```python
from build123d import *

# Parameters (mm, degrees)
SKETCH1_W           = 24.5
SKETCH1_H           = 13.110526316
SKETCH1_W_2         = 23.5
SKETCH1_H_2         = 10
BOSS_EXTRUDE1_DEPTH = 6
BOSS_EXTRUDE2_DEPTH = 6
SKETCH3_W           = 13.982681085
SKETCH3_H           = 4.437803864
CUT_EXTRUDE1_DEPTH  = 11
SKETCH4_W           = 0.982681085
SKETCH4_H           = 2.509369157
BOSS_EXTRUDE3_DEPTH = 6
SKETCH5_W           = 4.892282449
SKETCH5_H           = 6
BOSS_EXTRUDE4_DEPTH = 3.3
FILLET1_R           = 1.5
SKETCH6_W           = 3.982650634
SKETCH6_H           = 6.804776745
CUT_EXTRUDE2_DEPTH  = 10


with BuildPart() as part:
    # Sketch1 → Boss-Extrude1 (new body)
    with BuildSketch(Plane(origin=(0, 0, 0), x_dir=(1, 0, 0), z_dir=(0, 1, 0))):
        with Locations((-3.853684211, 3.800526316)):
            Rectangle(SKETCH1_W, SKETCH1_H)
        with Locations((-3.853684211, 3.855789474)):
            Rectangle(SKETCH1_W_2, SKETCH1_H_2, mode=Mode.SUBTRACT)
    extrude(amount=BOSS_EXTRUDE1_DEPTH)

    # Sketch2 → Boss-Extrude2 (add)
    with BuildSketch(Plane(origin=(0, 6, 0), x_dir=(1, 0, 0), z_dir=(0, 1, 0))):
        Polygon((-10.353684211, 10.355789474), (-10.353684211, 15.855789474), (2.646315789, 15.855789474), (2.646315789, 10.355789474), (4.146315789, 10.355789474), (4.146315789, 17.610127639), (-11.853684211, 17.610127639), (-11.853684211, 10.355789474), align=None)
    extrude(amount=-BOSS_EXTRUDE2_DEPTH)

    # Sketch3 → Cut-Extrude1 (cut)
    with BuildSketch(Plane(origin=(0, 6, 0), x_dir=(1, 0, 0), z_dir=(0, 1, 0))):
        with Locations((-3.362343669, 9.146256699)):
            Rectangle(SKETCH3_W, SKETCH3_H)
    extrude(amount=-CUT_EXTRUDE1_DEPTH, mode=Mode.SUBTRACT)

    # Sketch4 → Boss-Extrude3 (add)
    with BuildSketch(Plane(origin=(0, 6, 0), x_dir=(1, 0, 0), z_dir=(0, 1, 0))):
        with Locations((3.137656332, 10.110474052)):
            Rectangle(SKETCH4_W, SKETCH4_H)
    extrude(amount=-BOSS_EXTRUDE3_DEPTH)

    # Sketch5 → Boss-Extrude4 (add)
    with BuildSketch(Plane(origin=(8.396315789, 0, 0), x_dir=(0, 0, -1), z_dir=(1, 0, 0))):
        with Locations((7.90964825, 3)):
            Rectangle(SKETCH5_W, SKETCH5_H)
    extrude(amount=BOSS_EXTRUDE4_DEPTH)

    # Fillet1
    fillet1_edges = [part.edges().sort_by_distance(p)[0] for p in [
        (8.396315789, 3, -5.463507025),
    ]]
    fillet(fillet1_edges, radius=FILLET1_R)

    # Sketch6 → Cut-Extrude2 (cut)
    with BuildSketch(Plane(origin=(0, 6, 0), x_dir=(1, 0, 0), z_dir=(0, 1, 0))):
        with Locations((10.294706848, 7.545396136)):
            Rectangle(SKETCH6_W, SKETCH6_H)
    extrude(amount=-CUT_EXTRUDE2_DEPTH, mode=Mode.SUBTRACT)


solid = part.part
```
Check sheet for the modelled part. Datum: model origin and axes. Units: mm. A direction names the side the tool comes from. Coordinates: 2 decimals unless noted, no trailing zeros. Write each loop counter-clockwise with the first axis right and the second up, starting at its lowest first coordinate (ties: lowest second). Pieces come first, ordered by that corner, then holes. Notation, with made-up numbers: M -22,68.25 L 25,68.25 A26 cw 25,105.25 Z; hole C 58,47.5 d4. An arc over 180 degrees is marked long. Write item = value, one per line. Start each with the question number.
1. Go/stop test with flat-tipped pins: pin 1 (1.8 mm diameter, centred on y = 1.5, z = -6.5, fed in from +X); pin 2 (1.2 mm diameter, centred on x = 5.5, y = 2, fed in from -Z); pin 3 (3 mm diameter, centred on y = 2, z = 0.5, fed in from +X). Record where each tip stops, or that it passes through.
2. Mould release check, pull along X, two halves, no side actions. Record for faces 4 (the flat face through (-16.104, 3, -4)), 5 (the flat face through (-15.604, 3, -4)), 6 (the flat face through (6, 3, -10.356)): pulls with the +X half, pulls with the -X half, needs draft (parallel to the pull), parting line crosses it, or undercut.
3. Sectioned sample at B-B (z = -14.75). Record the cut outline in (x, y).
4. Thickness scan on probe 1 along Z at (x, y) = (-9.5, 3.35); probe 2 along X at (y, z) = (2.6, -7.5); probe 3 along X at (y, z) = (2.95, -11.75). Record the ranges inside material, lowest first.
5. Sectioned sample at C-C (y = 1.15). Record the cut outline in (x, z), then the cut area to 3 significant figures.
6. Sectioned sample at A-A (x = 3.25). Record the cut outline in (y, z), then the cut area to 3 significant figures.
7. Tool access check on faces 1 (the flat face through (4.146, 3, -14)), 2 (the flat face through (-11.854, 3, -14)), 3 (the flat face through (-4, 3, -15.856)). Record the directions out of +Z, -Z, +X, -X, +Y, -Y that give a thin tool (end or side, any length) a straight path to the whole face; none if there is none.
The answers:
q1.pin_1 = 8.3
q1.pin_2 = -10.36
q1.pin_3 = 8.4
q2.face_4 = pulls with the -X half
q2.face_5 = undercut
q2.face_6 = needs draft
q3.outline = M -11.85,0 L -10.35,0 L -10.35,6 L -11.85,6 Z; M 2.65,0 L 4.15,0 L 4.15,6 L 2.65,6 Z
q4.probe_1 = -17.61 to -15.86, 1.14 to 2.75
q4.probe_2 = -16.1 to -15.6, 7.9 to 8.3
q4.probe_3 = -11.85 to -10.35, 2.65 to 4.15
q5.outline = M -16.1,-10.36 L -11.85,-10.36 L -11.85,-17.61 L 4.15,-17.61 L 4.15,-10.36 L 8.3,-10.36 L 8.3,-4.14 L 8.41,-4.14 A1.5 cw 8.4,-3.96 L 8.4,2.75 L -16.1,2.75 Z; hole M -15.6,-8.86 L -10.35,-8.86 L -10.35,-15.86 L 2.65,-15.86 L 2.65,-8.86 L 7.9,-8.86 L 7.9,1.14 L -15.6,1.14 Z
q5.area = 111 mm²
q6.outline = M 0,-17.61 L 6,-17.61 L 6,-8.86 L 0,-8.86 Z; M 0,1.14 L 6,1.14 L 6,2.75 L 0,2.75 Z
q6.area = 62.2 mm²
q7.face_1 = -Z, +X, +Y, -Y
q7.face_2 = -Z, -X, +Y, -Y
q7.face_3 = +Y, -Y
